Here's how the part is built. I have some questions about the finished solid (model axes, mm). Face numbers are marked on the shaded views. A direction names the side the tool comes from. Round coordinates to 2 decimals unless told otherwise and drop trailing zeros. Write each loop counter-clockwise with the first axis right and the second up, starting at its lowest first coordinate (ties: lowest second). Pieces come first, ordered by that corner, then holes. Notation, with made-up numbers: (82, 9) - (136, 9) arc R6 ccw to (136, 15) - close; hole circle Ø7 at (51.25, -24.75). An arc over 180 degrees is marked (long way). One line per item, written item: value. Start each with the question number.
Item 1: For the marked faces 1 and 2, which set-ups out of +Z, -Z, +X, -X, +Y, -Y let a thin tool reach every point of the face, with its end or its side?
Item 2: Imagine slicing it at D-D, the plane z = 8.5. Please give me the cut outline in (x, y).
Item 3: If I drill on line 1 (Y direction, x = -15, z = 14.5); line 2 (X direction, y = 8.5, z = 3); line 3 (Y direction, x = -15, z = 15.5), over which ranges is the centre line in solid material (lowest first)?
Item 4: For P1, Ø1.8, axis at x = 15.5, y = 10, coming from the +Z side; P2, Ø2.5, axis at x = 15, y = 8.5, coming from the +Z side; P3, Ø6.5, axis at x = 13, y = 0, coming from the +Z side, each with a flat end and sliding along its axis, tell me the tip position at first contact or that it passes through.
Item 5: Imagine slicing it at A-A, the plane y = 0. Please give me the cut outline in (x, z), then the cut area to 3 significant figures.
Item 6: Imagine slicing it at C-C, the plane y = 8.5. Please give me the cut outline in (x, z).
Item 7: Imagine slicing it at B-B, the plane x = -7. Please give me the cut outline in (y, z).
Item 8: Thinking about a two-plate mould opening in X: for the marked faces 3, 4, 5 and 6, which applies, released by +X, released by -X, zero draft, split by the parting line, or undercut?
```python
from build123d import *

# Parameters (mm, degrees)
SKIZZE1_R                       = 1.5
AUFSATZ_LINEAR_AUSTRAGEN1_DEPTH = 16
SCHNITT_LINEAR_AUSTRAGEN1_DEPTH = 2
SKIZZE3_R                       = 2.5
SCHNITT_LINEAR_AUSTRAGEN2_DEPTH = 28.540878708
SKIZZE4_R                       = 3.05
SCHNITT_LINEAR_AUSTRAGEN3_DEPTH = 2.1
VERRUNDUNG1_R                   = 1


with BuildPart() as part:
    # Skizze1 → Aufsatz-Linear austragen1 (new body)
    with BuildSketch(Plane.XY):
        with BuildLine():
            Line((-16.1, 13.5), (16.1, 13.5))
            ThreePointArc((16.1, 13.5), (18.504163056, 12.504163056), (19.5, 10.1))
            Line((19.5, 10.1), (19.5, -10.1))
            ThreePointArc((19.5, -10.1), (18.504163056, -12.504163056), (16.1, -13.5))
            Line((16.1, -13.5), (-16.1, -13.5))
            ThreePointArc((-16.1, -13.5), (-18.504163056, -12.504163056), (-19.5, -10.1))
            Line((-19.5, -10.1), (-19.5, 10.1))
            ThreePointArc((-19.5, 10.1), (-18.504163056, 12.504163056), (-16.1, 13.5))
        make_face()
        with Locations((15, 8.5)):
            Circle(SKIZZE1_R, mode=Mode.SUBTRACT)
        with Locations((-15, -8.5)):
            Circle(SKIZZE1_R, mode=Mode.SUBTRACT)
    extrude(amount=AUFSATZ_LINEAR_AUSTRAGEN1_DEPTH)

    # Skizze2 → Schnitt-Linear austragen1 (cut)
    with BuildSketch(Plane.XY.offset(16)):
        with BuildLine():
            Line((-15, 4.5), (15, 4.5))
            ThreePointArc((15, 4.5), (16.414213562, 3.914213562), (17, 2.5))
            Line((17, 2.5), (17, -2.5))
            ThreePointArc((17, -2.5), (16.414213562, -3.914213562), (15, -4.5))
            Line((15, -4.5), (-15, -4.5))
            ThreePointArc((-15, -4.5), (-16.414213562, -3.914213562), (-17, -2.5))
            Line((-17, -2.5), (-17, 2.5))
            ThreePointArc((-17, 2.5), (-16.414213562, 3.914213562), (-15, 4.5))
        make_face()
    extrude(amount=-SCHNITT_LINEAR_AUSTRAGEN1_DEPTH, mode=Mode.SUBTRACT)

    # Skizze3 → Schnitt-Linear austragen2 (cut, through all)
    with BuildSketch(Plane.XY.offset(14)):
        with Locations((-13, 0)):
            Circle(SKIZZE3_R)
        with Locations(Location((13, 0, 0), (0, 0, 180))):
            Circle(SKIZZE3_R)
    extrude(amount=-SCHNITT_LINEAR_AUSTRAGEN2_DEPTH, mode=Mode.SUBTRACT)

    # Skizze4 → Schnitt-Linear austragen3 (cut)
    with BuildSketch(Plane.XY.offset(16)):
        with Locations((15, 8.5)):
            Circle(SKIZZE4_R)
        with Locations((-15, -8.5)):
            Circle(SKIZZE4_R)
    extrude(amount=-SCHNITT_LINEAR_AUSTRAGEN3_DEPTH, mode=Mode.SUBTRACT)

    # Verrundung1
    verrundung1_edges = [part.edges().sort_by_distance(p)[0] for p in [
        (-18.504163056, 12.504163056, 16),
        (-19.5, 0, 16),
        (-18.504163056, -12.504163056, 16),
        (0, -13.5, 16),
        (18.504163056, -12.504163056, 16),
        (19.5, 0, 16),
        (18.504163056, 12.504163056, 16),
        (0, 13.5, 16),
    ]]
    fillet(verrundung1_edges, radius=VERRUNDUNG1_R)


solid = part.part
```
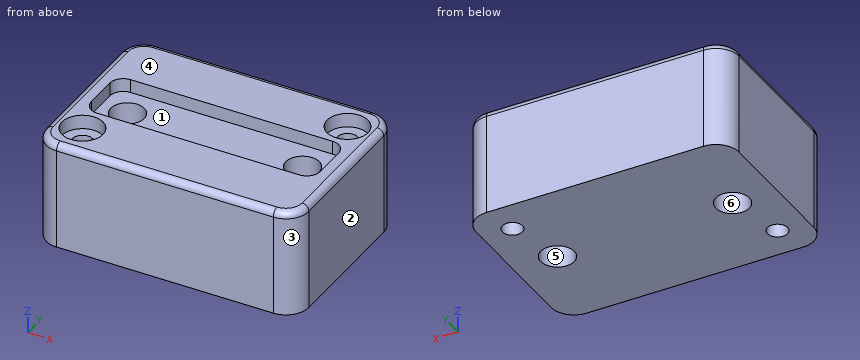
Values follow:
1. face 1: +Z
1. face 2: +Z, -Z, +X, +Y, -Y
2. outline: (-19.5, -10.1) arc R3.4 ccw to (-16.1, -13.5) - (16.1, -13.5) arc R3.4 ccw to (19.5, -10.1) - (19.5, 10.1) arc R3.4 ccw to (16.1, 13.5) - (-16.1, 13.5) arc R3.4 ccw to (-19.5, 10.1) - close; hole circle Ø3 at (-15, -8.5); hole circle Ø5 at (-13, 0); hole circle Ø5 at (13, 0); hole circle Ø3 at (15, 8.5)
3. line 1: y = -13.5 to -11.55, -5.45 to -4.5, 4.5 to 13.5
3. line 2: x = -19.5 to 13.5, 16.5 to 19.5
3. line 3: y = -13.37 to -11.55, -5.45 to -4.5, 4.5 to 13.37
4. P1: stops at z = 13.9
4. P2: passes through
4. P3: stops at z = 14
5. outline: (-19.5, 0) - (-15.5, 0) - (-15.5, 14) - (-17, 14) - (-17, 16) - (-18.5, 16) arc R1 ccw to (-19.5, 15) - close; (-10.5, 0) - (10.5, 0) - (10.5, 14) - (-10.5, 14) - close; (15.5, 0) - (19.5, 0) - (19.5, 15) arc R1 ccw to (18.5, 16) - (17, 16) - (17, 14) - (15.5, 14) - close
5. area: 416 mm^2
6. outline: (-19.5, 0) - (13.5, 0) - (13.5, 13.9) - (11.95, 13.9) - (11.95, 16) - (-18.5, 16) arc R1 ccw to (-19.5, 15) - close; (16.5, 0) - (19.5, 0) - (19.5, 15) arc R1 ccw to (18.5, 16) - (18.05, 16) - (18.05, 13.9) - (16.5, 13.9) - close
7. outline: (-13.5, 0) - (13.5, 0) - (13.5, 15) arc R1 ccw to (12.5, 16) - (4.5, 16) - (4.5, 14) - (-4.5, 14) - (-4.5, 16) - (-12.5, 16) arc R1 ccw to (-13.5, 15) - close
8. face 3: released by +X
8. face 4: zero draft
8. face 5: undercut
8. face 6: undercut
